Check sheet for the drawn part. Datum: minimum x, y, z corner. Units: mm. A direction names the side the tool comes from. Round coordinates to 2 decimals unless told otherwise and drop trailing zeros. Order: outer loops, then holes, each group sorted by start corner. A loop starts at its lowest first (then second) coordinate and runs counter-clockwise, first axis right, second up. Notation, with made-up numbers: (14, -16) -> (73, -16) arc R26 cw to (73, 11) -> close; hole circle Ø11 at (58.25, 64.25). An arc over 180 degrees is marked (long way). Use CSV: the item, a comma, the result in double quotes.
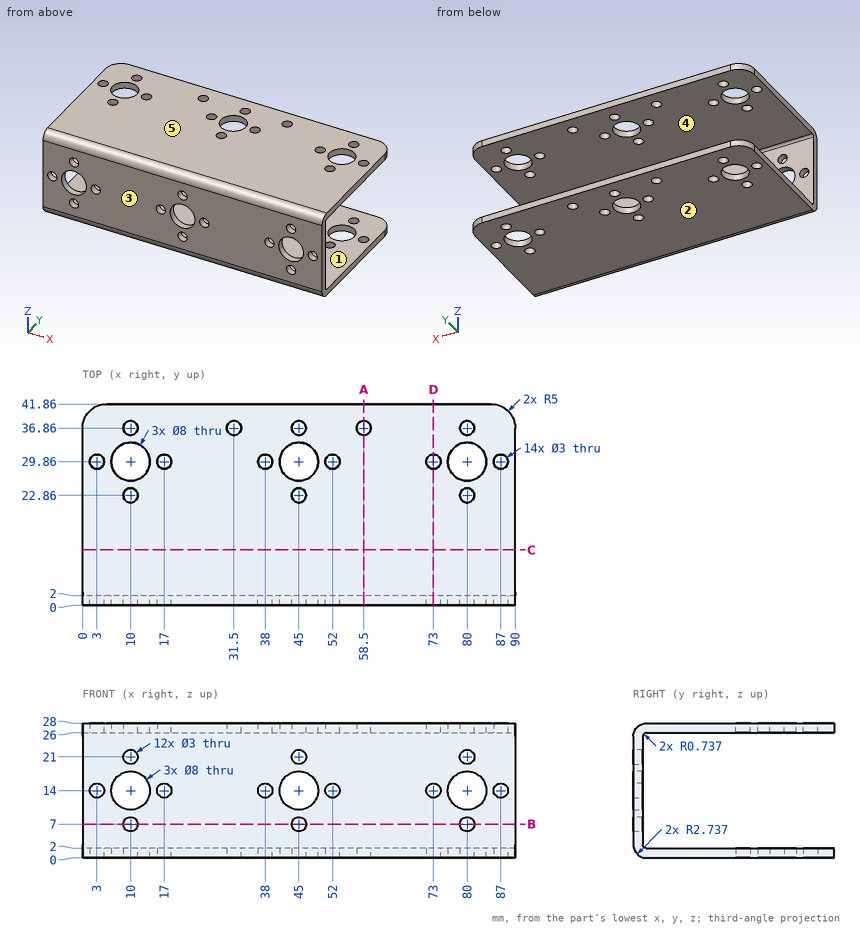
Q1. Go/stop test with flat-tipped pins: pin 1 (1.8 mm diameter, centred on x = 17, y = 29.86, fed in from -Z); pin 2 (4 mm diameter, centred on x = 45, z = 21, fed in from +Y). Record where each tip stops, or that it passes through.
Result sheet:
pin 1,"passes through"
pin 2,"stops at y = 2"
Q2. Sectioned sample at D-D, the plane x = 73. Enter the section's corners in (y, z).
Result sheet:
outline,"(0, 2.74) arc R2.74 ccw to (2.74, 0) -> (28.36, 0) -> (28.36, 2) -> (2.74, 2) arc R0.74 cw to (2, 2.74) -> (2, 12.5) -> (0, 12.5) -> close; (0, 15.5) -> (2, 15.5) -> (2, 25.26) arc R0.74 cw to (2.74, 26) -> (28.36, 26) -> (28.36, 28) -> (2.74, 28) arc R2.74 ccw to (0, 25.26) -> close; (31.36, 0) -> (41.86, 0) -> (41.86, 2) -> (31.36, 2) -> close; (31.36, 26) -> (41.86, 26) -> (41.86, 28) -> (31.36, 28) -> close"
Q3. Access from +Z, -Z, +X, -X, +Y, -Y to the whole of each face (thin tool, end or side, straight path). Record for the marked faces 1 and 2.
Result sheet:
face 1,"+X, -X, +Y"
face 2,"-Z, +X, -X, +Y, -Y"
Q4. Mould release check, pull along Z, two halves, no side actions. Record for the marked faces 3, 4 and 5: pulls with the +Z half, pulls with the -Z half, needs draft (parallel to the pull), parting line crosses it, or undercut.
Result sheet:
face 3,"needs draft"
face 4,"undercut"
face 5,"pulls with the +Z half"
Q5. Sectioned sample at C-C, the plane y = 11.5. Enter the section's corners in (x, z), then the cut area to 3 significant figures.
Result sheet:
outline,"(0, 0) -> (90, 0) -> (90, 2) -> (0, 2) -> close; (0, 26) -> (90, 26) -> (90, 28) -> (0, 28) -> close"
area,"360 mm^2"
Q6. Sectioned sample at A-A, the plane x = 58.5. Enter the section's corners in (y, z).
Result sheet:
outline,"(0, 2.74) arc R2.74 ccw to (2.74, 0) -> (35.36, 0) -> (35.36, 2) -> (2.74, 2) arc R0.74 cw to (2, 2.74) -> (2, 25.26) arc R0.74 cw to (2.74, 26) -> (35.36, 26) -> (35.36, 28) -> (2.74, 28) arc R2.74 ccw to (0, 25.26) -> close; (38.36, 0) -> (41.86, 0) -> (41.86, 2) -> (38.36, 2) -> close; (38.36, 26) -> (41.86, 26) -> (41.86, 28) -> (38.36, 28) -> close"
Q7. Sectioned sample at B-B, the plane z = 7. Enter the section's corners in (x, y), then the cut area to 3 significant figures.
Result sheet:
outline,"(0, 0) -> (8.5, 0) -> (8.5, 2) -> (0, 2) -> close; (11.5, 0) -> (43.5, 0) -> (43.5, 2) -> (11.5, 2) -> close; (46.5, 0) -> (78.5, 0) -> (78.5, 2) -> (46.5, 2) -> close; (81.5, 0) -> (90, 0) -> (90, 2) -> (81.5, 2) -> close"
area,"162 mm^2"
Q8. Scan lines: L1, parallel to X at y = 0.8, z = 7; L2, parallel to Z at x = 79.5, y = 11; L3, parallel to Y at x = 80, z = 1.3. Record each from-to range of solid material in increasing order.
Result sheet:
L1,"x = 0 to 8.5, 11.5 to 43.5, 46.5 to 78.5, 81.5 to 90"
L2,"z = 0 to 2, 26 to 28"
L3,"y = 0.41 to 21.36, 24.36 to 25.86, 33.86 to 35.36, 38.36 to 41.86"
